Check sheet for the modelled part. Datum: model origin and axes. Units: mm. Give positions to 0.01 mm unless a question says otherwise; leave off trailing zeros. Order: outer loops, then holes, each group sorted by start corner. A loop starts at its lowest first (then second) coordinate and runs counter-clockwise, first axis right, second up. Notation, with made-up numbers: (3.5, -13.75) -> (40.5, -13.75) arc R9 cw to (40.5, -8.75) -> close; hole circle Ø11 at (-36, 76). An arc over 180 degrees is marked (long way). Answer in a Markdown table with one row per item. Add a question column.
(1) Thickness scan on L1, parallel to X at y = -23, z = 4.5; L2, parallel to Y at x = 0.5, z = 4.25; L3, parallel to Z at x = -6, y = -43.5. Record the ranges inside material, lowest first. Write a range as [from, to].
(2) Cross-section at B-B (z = -8.5). Record the cut outline in (x, y), then the cut area to 3 significant figures.
(3) Cross-section at A-A (y = -39). Record the cut outline in (x, z).
(4) Cross-section at C-C (x = -7.5). Record the cut outline in (y, z), then the cut area to 3 significant figures.
(5) Release check for a two-part mould opening along Y. For faces 1 (the face through (0, -50, 0)), 2 (the face through (-4.061, -24.042, 2.503)), 3 (the face through (6.053, -24.65, 1.355)), 4 (the face through (0, 0, 0)) record: released by +Y, released by -Y, zero draft, split by the parting line, or undercut.
(6) Go/stop test with flat-tipped pins: pin 1 (4 mm diameter, centred on x = -3.5, y = -11.5, fed in from +Z); pin 2 (4 mm diameter, centred on y = -39, z = -4.5, fed in from -X); pin 3 (4 mm diameter, centred on y = -6, z = -5.5, fed in from +X). Record where each tip stops, or that it passes through.
```python
from build123d import *

# Parameters (mm, degrees)
F1_DEPTH = 50
F2_R     = 3
F5_DEPTH = 9.24953
F3_R     = 2
F6_DEPTH = 10.30413
F4_R     = 1.5
F7_DEPTH = 9.13494


with BuildPart() as f1:
    # F0 (on Front) → F1 (new body)
    with BuildSketch(Plane.XZ):
        Polygon((-9.2966205801, 5.7323870165), (-0.6050675001, -9.6636938179), (8.7033765413, 5.7425669072), align=None)
    extrude(amount=F1_DEPTH)

    # F2 (on face) → F5 (cut)
    with BuildSketch(Plane(origin=(3.8340726786, 0, -2.3165420615), x_dir=(0, 1, 0), z_dir=(0.8559033736, 0, -0.5171357801))):
        with Locations((-24, 0)):
            Circle(F2_R)
    extrude(amount=-F5_DEPTH, mode=Mode.SUBTRACT)

    # F3 (on face) → F6 (cut)
    with BuildSketch(Plane(origin=(-0.0032449215, 0, 5.7376428811), x_dir=(0.9999998401, 0, 0.0005655495), z_dir=(-0.0005655495, 0, 0.9999998401))):
        with Locations((0, -24)):
            Circle(F3_R)
    extrude(amount=-F6_DEPTH, mode=Mode.SUBTRACT)

    # F4 (on face) → F7 (cut)
    with BuildSketch(Plane(origin=(-4.5958448678, 0, -2.5944933678), x_dir=(0, -1, 0), z_dir=(-0.8708190517, 0, -0.491603681))):
        with Locations((24, 0)):
            Circle(F4_R)
    extrude(amount=-F7_DEPTH, mode=Mode.SUBTRACT)


solid = f1.part
```
Answer below:
| question | item | result |
|---|---|---|
| 1 | L1 | x = [-8.6, -2.85], [-1.98, -1.73], [1.73, 7.95] |
| 1 | L2 | y = [-50, -25.94], [-22.06, 0] |
| 1 | L3 | z = [-0.11, 5.73] |
| 2 | outline | (-1.26, -50) -> (0.1, -50) -> (0.1, 0) -> (-1.26, 0) -> close |
| 2 | area | 68.0 mm² |
| 3 | outline | (-9.3, 5.73) -> (-0.61, -9.66) -> (8.7, 5.74) -> close |
| 4 | outline | (-50, 2.55) -> (0, 2.55) -> (0, 5.73) -> (-50, 5.73) -> close |
| 4 | area | 159 mm² |
| 5 | face 1 | released by -Y |
| 5 | face 2 | undercut |
| 5 | face 3 | zero draft |
| 5 | face 4 | released by +Y |
| 6 | pin 1 | stops at z = 5.74 |
| 6 | pin 2 | stops at x = -4.65 |
| 6 | pin 3 | stops at x = 3.12 |
